Check sheet for the drawn part. Datum: minimum x, y, z corner. Units: mm. A direction names the side the tool comes from. Give positions to 0.01 mm unless a question says otherwise; leave off trailing zeros. Order: outer loops, then holes, each group sorted by start corner. A loop starts at its lowest first (then second) coordinate and runs counter-clockwise, first axis right, second up. Notation, with made-up numbers: M 89,62 L 135,62 A32 cw 135,93 Z; hole C 6,-1.5 d9. An arc over 180 degrees is marked long. Put each result on its own line as item: value. Start each with the question number.
Q1. Material ranges on L1, parallel to X at y = 39, z = 47; L2, parallel to Y at x = 20, z = 36; L3, parallel to X at y = 19.5, z = 23.5, recorded low to high.
Q2. Access from +Z, -Z, +X, -X, +Y, -Y to the whole of each face (thin tool, end or side, straight path). Record for the marked faces 4, 5 and 6.
Q3. Section check A-A on x = 50. Record the cut outline in (y, z) (1 decimal), then the cut area to 3 significant figures.
Q4. Section check D-D on y = 230. Record the cut outline in (x, z), then the cut area to 3 significant figures.
Q5. Section check B-B on y = 22.5. Record the cut outline in (x, z) (1 decimal), then the cut area to 3 significant figures.
Q6. Mould release check, pull along Z, two halves, no side actions. Record for the marked faces 1, 2 and 3: +Z half, -Z half, draft (parallel to the pull), parting line (faces both ways), or undercut.
Q7. Go/stop test with flat-tipped pins: pin 1 (5 mm diameter, centred on x = 39, y = 43.5, fed in from -Z); pin 2 (16 mm diameter, centred on y = 230, z = 50, fed in from -X); pin 3 (8 mm diameter, centred on y = 91.5, z = 26, fed in from +X). Record where each tip stops, or that it passes through.
Q8. Section check C-C on z = 11. Record the cut outline in (x, y), then the cut area to 3 significant figures.
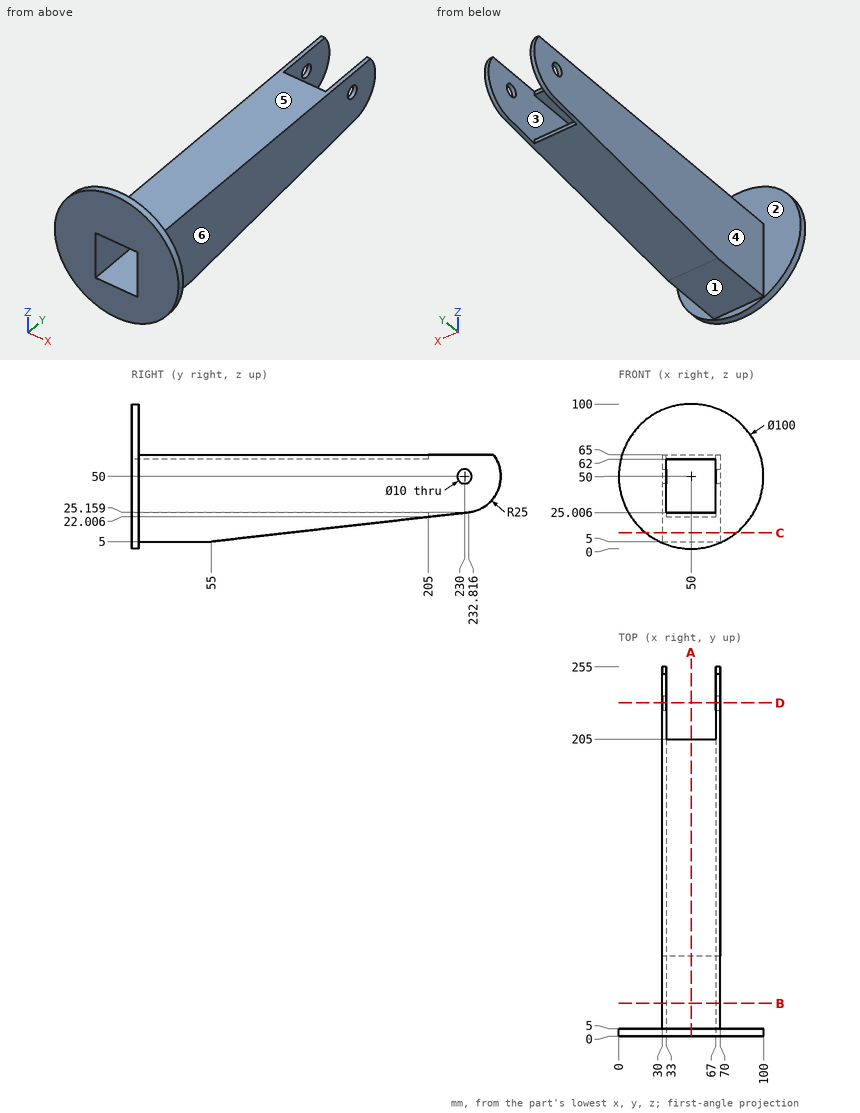
Results found:
1. L1: x = 30 to 33, 67 to 70
1. L2: y = 0 to 5
1. L3: x = 30 to 70
2. face 4: +Z, -Z, -X, +Y
2. face 5: +Z, +X, -X, +Y
2. face 6: +Z, -Z, +X, +Y
3. outline: M 0,0 L 5,0 L 5,5 L 55,5 L 205,22 L 205,25 L 0,25 Z; M 0,62 L 205,62 L 205,65 L 5,65 L 5,100 L 0,100 Z
3. area: 3,640 mm^2
4. outline: M 30,24.84 L 33,24.84 L 33,45 L 30,45 Z; M 30,55 L 33,55 L 33,65 L 30,65 Z; M 67,24.84 L 70,24.84 L 70,45 L 67,45 Z; M 67,55 L 70,55 L 70,65 L 67,65 Z
4. area: 181 mm^2
5. outline: M 30,5 L 70,5 L 70,65 L 30,65 Z; hole M 33,25 L 67,25 L 67,62 L 33,62 Z
5. area: 1,140 mm^2
6. face 1: -Z half
6. face 2: draft
6. face 3: undercut
7. pin 1: stops at z = 5
7. pin 2: stops at x = 30
7. pin 3: stops at x = 70
8. outline: M 18.71,0 L 81.29,0 L 81.29,5 L 70,5 L 70,107.92 L 30,107.92 L 30,5 L 18.71,5 Z
8. area: 4,430 mm^2
